Geometry: final body of the model. Coordinates: model frame, mm. A direction names the side the tool comes from. Coordinates: 2 decimals unless noted, no trailing zeros. Loops run counter-clockwise (first coordinate to the right, second up) from the corner with the lowest first, then second, coordinate; pieces in that order, holes last. Notation, with made-up numbers: (51.5, -39) - (93.5, -39) arc R18 cw to (93.5, -14) - close; hole circle Ø1 at (69.25, 46). An arc over 180 degrees is marked (long way). Put each result on its own line as item: value. Start each with the question number.
1) Section D-D on x = -9.5. Output: boundary loops of the cut face in (y, z), and give its area (3 significant figures).
2) Section B-B on z = 7.25. Output: boundary loops of the cut face in (x, y), and give its area (3 significant figures).
3) Reachability of faces 5 (the flat face through (-20, -2, 8)), 6 (the cylindrical face through (12.586, 0.066, 3.113)), 7 (the cylindrical face through (-1.126, 3.983, 8.097)) from +Z, -Z, +X, -X, +Y, -Y: full face, straight path, thin tool, end or side. Return the list, or none.
4) Contact query for flat-ended pins moving along their axis: pin 1 Ø2.5 at (x, y) = (14.08, 0) entering from +Z; pin 2 Ø5 at (x, y) = (-9.92, 0) entering from -Z; pin 3 Ø4.5 at (x, y) = (-5.5, 0.5) entering from +Z. Output: stop coordinate, or through.
5) Section C-C on z = 5.25. Output: boundary loops of the cut face in (x, y).
6) Section A-A on y = 0. Output: boundary loops of the cut face in (x, z).
7) Draft query along Y for faces 1 (the cylindrical face through (18.215, -0.077, 8.097)), 2 (the flat face through (0, 0, 0)), 3 (the flat face through (0, 12.2, 5)), 4 (the flat face through (9, 3.5, 8)). Return one class per face: +Y half, -Y half, draft (parallel to the pull), parting line (faces both ways), or undercut.
8) Material intervals for line 1 along Y through (x, z) = (13, 6.75); line 2 along X through (y, z) = (-1.25, 2.5); line 3 along Y through (x, z) = (-19.5, 6.75), sorted ascending. Write a range as from..to.
```python
from build123d import *

# Parameters (mm, degrees)
SKETCH2_W           = 24.4
SKETCH2_H           = 45
BOSS_EXTRUDE1_DEPTH = 10
CUT_EXTRUDE1_DEPTH  = 3.86
SKETCH4_R           = 1.5
CUT_EXTRUDE2_DEPTH  = 27.320896641
CUT_EXTRUDE4_DEPTH  = 3.86


with BuildPart() as part:
    # Sketch2 → Boss-Extrude1 (new body)
    with BuildSketch(Plane(origin=(0, 0, 0), x_dir=(0, 1, 0), z_dir=(0, 0, 1))):
        Rectangle(SKETCH2_W, SKETCH2_H)
    extrude(amount=BOSS_EXTRUDE1_DEPTH)

    # Sketch3 → Cut-Extrude1 (cut)
    with BuildSketch(Plane.XY.offset(10)):
        with BuildLine():
            Line((14.715504893, 3.5), (2.384966333, 3.5))
            ThreePointArc((2.384966333, 3.5), (-1.174243063, 3.996719292), (-4.461463541, 5.448918697))
            ThreePointArc((-4.461463541, 5.448918697), (-17.115033667, 0), (-4.461463541, -5.448918697))
            ThreePointArc((-4.461463541, -5.448918697), (-1.174243063, -3.996719292), (2.384966333, -3.5))
            Line((2.384966333, -3.5), (14.715504893, -3.5))
            ThreePointArc((14.715504893, -3.5), (18.215504893, 0), (14.715504893, 3.5))
        make_face()
    extrude(amount=-CUT_EXTRUDE1_DEPTH, mode=Mode.SUBTRACT)

    # Sketch4 → Cut-Extrude2 (cut, through all)
    with BuildSketch(Plane.XY.offset(6.14)):
        with Locations((10.084966333, 0)):
            Circle(SKETCH4_R)
        with Locations((14.084966333, 0)):
            Circle(SKETCH4_R)
        with Locations((-9.915033667, 0)):
            Circle(SKETCH4_R)
    extrude(amount=-CUT_EXTRUDE2_DEPTH, mode=Mode.SUBTRACT)

    # Sketch6 → Cut-Extrude4 (cut)
    with BuildSketch(Plane.XY.offset(10)):
        with BuildLine():
            Line((-22.5, 2), (-16.843449814, 2))
            ThreePointArc((-16.843449814, 2), (-17.115033667, 0), (-16.843449814, -2))
            Line((-16.843449814, -2), (-22.5, -2))
            Line((-22.5, -2), (-22.5, 2))
        make_face()
    extrude(amount=-CUT_EXTRUDE4_DEPTH, mode=Mode.SUBTRACT)


solid = part.part
```
Answer block:
1. outline: (-12.2, 0) - (-1.44, 0) - (-1.44, 6.14) - (-7.5, 6.14) - (-7.5, 10) - (-12.2, 10) - close; (1.44, 0) - (12.2, 0) - (12.2, 10) - (7.5, 10) - (7.5, 6.14) - (1.44, 6.14) - close
1. area: 168 mm²
2. outline: (-22.5, -12.2) - (22.5, -12.2) - (22.5, 12.2) - (-22.5, 12.2) - (-22.5, 2) - (-16.84, 2) arc R7.5 cw to (-4.46, 5.45) arc R13 ccw to (2.38, 3.5) - (14.72, 3.5) arc R3.5 cw to (14.72, -3.5) - (2.38, -3.5) arc R13 ccw to (-4.46, -5.45) arc R7.5 cw to (-16.84, -2) - (-22.5, -2) - close
2. area: 755 mm²
3. face 5: +Z, -X
3. face 6: +Z, -Z
3. face 7: +Z
4. pin 1: passes through
4. pin 2: stops at z = 0
4. pin 3: stops at z = 6.14
5. outline: (-22.5, -12.2) - (22.5, -12.2) - (22.5, 12.2) - (-22.5, 12.2) - close; hole circle Ø3 at (-9.92, 0); hole circle Ø3 at (10.08, 0); hole circle Ø3 at (14.08, 0)
6. outline: (-22.5, 0) - (-11.42, 0) - (-11.42, 6.14) - (-22.5, 6.14) - close; (-8.42, 0) - (8.58, 0) - (8.58, 6.14) - (-8.42, 6.14) - close; (11.58, 0) - (12.58, 0) - (12.58, 6.14) - (11.58, 6.14) - close; (15.58, 0) - (22.5, 0) - (22.5, 10) - (18.22, 10) - (18.22, 6.14) - (15.58, 6.14) - close
7. face 1: undercut
7. face 2: draft
7. face 3: +Y half
7. face 4: undercut
8. line 1: y = -12.2..-3.5, 3.5..12.2
8. line 2: x = -22.5..-10.74, -9.09..9.26, 10.91..13.26, 14.91..22.5
8. line 3: y = -12.2..-2, 2..12.2
